Part model, mm, in its own coordinate system. Give positions to 0.01 mm unless a question says otherwise; leave off trailing zeros. Loops run counter-clockwise (first coordinate to the right, second up) from the corner with the lowest first, then second, coordinate; pieces in that order, holes last. Notation, with made-up numbers: (-10.75, -23.5) -> (-6.75, -23.5) arc R25 cw to (-6.75, -7.5) -> close; hole circle Ø8 at (30, 40). An arc over 180 degrees is marked (long way). One line per question, with ' | ' between items.
```python
from build123d import *

# Parameters (mm, degrees)
SKETCH1_R           = 1.3462
SKETCH1_W           = 5.4034
SKETCH1_H           = 22.6066
SKETCH1_W_2         = 60.6932
SKETCH1_H_2         = 7.81
SKETCH1_W_3         = 15.431
SKETCH1_H_3         = 21.4039
SKETCH1_W_4         = 31.9679
SKETCH1_H_4         = 18.2371
SKETCH1_W_5         = 5.588
SKETCH1_H_5         = 33.5001
BOSS_EXTRUDE1_DEPTH = 3.048


with BuildPart() as part:
    # Sketch1 → Boss-Extrude1 (new body)
    with BuildSketch(Plane.XY):
        with BuildLine():
            Line((40.325007375, 24.068294304), (61.214907375, 24.068294304))
            Line((61.214907375, 24.068294304), (61.214907375, 26.683892153))
            ThreePointArc((61.214907375, 26.683892153), (60.103884597, 29.386886916), (57.404932375, 30.507694304))
            Line((57.404932375, 30.507694304), (-34.084892625, 30.507694304))
            ThreePointArc((-34.084892625, 30.507694304), (-36.778969461, 29.391771141), (-37.894892625, 26.697694304))
            Line((-37.894892625, 26.697694304), (-37.894892625, -32.641005696))
            ThreePointArc((-37.894892625, -32.641005696), (-36.778969461, -35.335082532), (-34.084892625, -36.451005696))
            Line((-34.084892625, -36.451005696), (-23.844892625, -33.084405696))
            Line((-23.844892625, -33.084405696), (28.474307375, -33.084405696))
            Line((28.474307375, -33.084405696), (38.714307375, -36.451005696))
            Line((38.714307375, -36.451005696), (57.405007375, -36.451005696))
            ThreePointArc((57.405007375, -36.451005696), (60.108826144, -35.325305244), (61.214907375, -32.613401529))
            Line((61.214907375, -32.613401529), (61.214907375, -28.627805696))
            Line((61.214907375, -28.627805696), (35.575007375, -28.627805696))
            Line((35.575007375, -28.627805696), (35.575007375, -12.628005696))
            Line((35.575007375, -12.628005696), (56.975007375, -12.628005696))
            Line((56.975007375, -12.628005696), (56.975007375, -9.121805696))
            Line((56.975007375, -9.121805696), (40.325007375, -9.121805696))
            Line((40.325007375, -9.121805696), (40.325007375, 4.997894304))
            Line((40.325007375, 4.997894304), (56.975007375, 4.997894304))
            Line((56.975007375, 4.997894304), (56.975007375, 8.658194304))
            Line((56.975007375, 8.658194304), (40.325007375, 8.658194304))
            Line((40.325007375, 8.658194304), (40.325007375, 24.068294304))
        make_face()
        with Locations(Location((57.404932375, 26.697694304, 0), (0, 0, 180))):
            Circle(SKETCH1_R, mode=Mode.SUBTRACT)
        with Locations(Location((57.405007375, -32.641005696, 0), (0, 0, 180))):
            Circle(SKETCH1_R, mode=Mode.SUBTRACT)
        with Locations(Location((-34.084892625, -32.641005696, 0), (0, 0, 180))):
            Circle(SKETCH1_R, mode=Mode.SUBTRACT)
        with Locations(Location((-34.084892625, 26.697694304, 0), (0, 0, 180))):
            Circle(SKETCH1_R, mode=Mode.SUBTRACT)
        with Locations((16.546707375, -19.663505696)):
            Rectangle(SKETCH1_W, SKETCH1_H, mode=Mode.SUBTRACT)
        with Locations((1.341707375, 21.991994304)):
            Rectangle(SKETCH1_W_2, SKETCH1_H_2, mode=Mode.SUBTRACT)
        with Locations((25.156507375, 5.270444304)):
            Rectangle(SKETCH1_W_3, SKETCH1_H_3, mode=Mode.SUBTRACT)
        with Locations((-5.654942625, 1.475544304)):
            Rectangle(SKETCH1_W_4, SKETCH1_H_4, mode=Mode.SUBTRACT)
        with Locations((-26.210892625, -6.948855696)):
            Rectangle(SKETCH1_W_5, SKETCH1_H_5, mode=Mode.SUBTRACT)
    extrude(amount=BOSS_EXTRUDE1_DEPTH)


solid = part.part
```
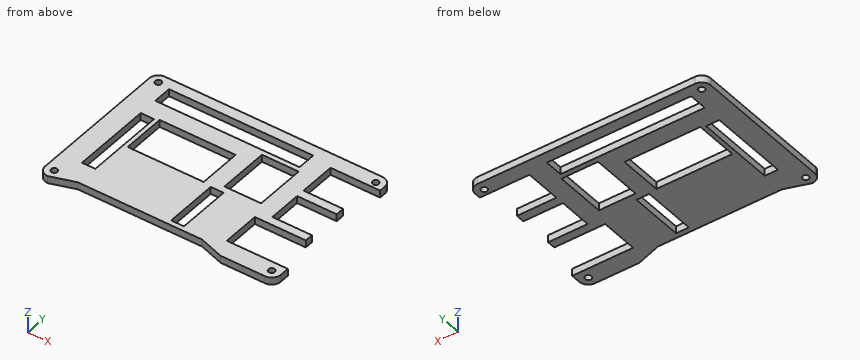
1) Saw through at C-C (y = 6). Give the cut face in (x, z) (3 decimals), and give its area (3 significant figures).
Found:
outline: (-37.895, 0) -> (-29.005, 0) -> (-29.005, 3.048) -> (-37.895, 3.048) -> close; (-23.417, 0) -> (-21.639, 0) -> (-21.639, 3.048) -> (-23.417, 3.048) -> close; (10.329, 0) -> (17.441, 0) -> (17.441, 3.048) -> (10.329, 3.048) -> close; (32.872, 0) -> (56.975, 0) -> (56.975, 3.048) -> (32.872, 3.048) -> close | area: 128 mm2
2) Saw through at B-B (x = -5). Give the cut face in (y, z).
Found:
outline: (-33.08, 0) -> (-7.64, 0) -> (-7.64, 3.05) -> (-33.08, 3.05) -> close; (10.59, 0) -> (18.09, 0) -> (18.09, 3.05) -> (10.59, 3.05) -> close; (25.9, 0) -> (30.51, 0) -> (30.51, 3.05) -> (25.9, 3.05) -> close
3) Saw through at A-A (y = -26.5). Give the cut face in (x, z) (3 decimals).
Found:
outline: (-37.895, 0) -> (13.845, 0) -> (13.845, 3.048) -> (-37.895, 3.048) -> close; (19.248, 0) -> (35.575, 0) -> (35.575, 3.048) -> (19.248, 3.048) -> close
4) Saw through at D-D (x = 51). Give the cut face in (y, z).
Found:
outline: (-36.45, 0) -> (-28.63, 0) -> (-28.63, 3.05) -> (-36.45, 3.05) -> close; (-12.63, 0) -> (-9.12, 0) -> (-9.12, 3.05) -> (-12.63, 3.05) -> close; (5, 0) -> (8.66, 0) -> (8.66, 3.05) -> (5, 3.05) -> close; (24.07, 0) -> (30.51, 0) -> (30.51, 3.05) -> (24.07, 3.05) -> close
5) Drill centre lines: line 1 (X direction, y = -16.5, z = 1.6) (3 decimals); line 2 (Y direction, x = 6.5, z = 2.6); line 3 (X direction, y = 6.5, z = 2.1) (3 decimals). Where is each one in solid material? Low to high.
Found:
line 1: -37.895 to -29.005, -23.417 to 13.845, 19.248 to 35.575 | line 2: -33.08 to -7.64, 10.59 to 18.09, 25.9 to 30.51 | line 3: -37.895 to -29.005, -23.417 to -21.639, 10.329 to 17.441, 32.872 to 56.975
6) Pin check, flat tips, straight feed: P1, Ø1.5, axis at x = -6.5, z = 1, coming from the -Y side; P2, Ø0.9, axis at x = -27, z = 1.5, coming from the -Y side; P3, Ø0.9, axis at y = -19, z = 1, coming from the +X side (3 decimals). Stop position of each tip, or through.
Found:
P1: y = -33.08 | P2: y = -34.27 | P3: x = 35.575
